Work out the finished part from the listing and answer in its coordinate system (mm). Face numbers are marked on the shaded views. A direction names the side the tool comes from. Round coordinates to 2 decimals unless told otherwise and drop trailing zeros. Order: outer loops, then holes, each group sorted by start corner. A loop starts at its lowest first (then second) coordinate and runs counter-clockwise, first axis right, second up. Notation, with made-up numbers: (-12.5, 27) -> (8.5, 27) arc R9 ccw to (8.5, 31) -> close; hole circle Ø7 at (50, 41). An arc over 180 degrees is marked (long way). Use a Markdown table: item, result. Add a question column.
Item 1: A cutting plane is placed at C-C, the plane z = 15. Determine the outline of the cut face in (x, y).
Item 2: A cutting plane is placed at A-A, the plane y = 0. Determine the outline of the cut face in (x, z), plus the area to 3 significant figures.
Item 3: Find the intervals of material crossed by L1, parallel to Z at x = 2, y = -0.75; L2, parallel to X at y = 5.25, z = 17.5; L3, parallel to Y at x = -6.75, z = 5.75, in increasing order. Write a range as [from, to].
Item 4: A tool of negligible diameter and unlimited length cuts with its end or side. For the marked faces 1, 2 and 3, from which of +Z, -Z, +X, -X, +Y, -Y can it reach the whole face along a straight path? Write none if from no direction.
Item 5: Flat-ended cylindrical pins translate along their axes: P1, Ø1.5, axis at y = -1.5, z = 12.5, coming from the +X side; P2, Ø2, axis at x = -3, z = -0.5, coming from the -Y side; P3, Ø2, axis at x = 2.5, z = 8.5, coming from the +Y side. Find the tip coordinate at first contact, or state that the pin passes through.
from build123d import *

# Parameters (mm, degrees)
BOSS_EXTRUDE1_START = 2
SKETCH2_R           = 1.25
BOSS_EXTRUDE1_DEPTH = 2


with BuildPart() as part:
    # Sketch1 → Revolve1 (revolve)
    with BuildSketch(Plane(origin=(0, 0, 0), x_dir=(1, 0, 0), z_dir=(0, 1, 0))):
        Polygon((1.25, 1.9), (0, 1.9), (0, -22.7), (0.8476, -22.7), (1, -22.5476), (1, -18.7), (9.125906359, -18.7), (10.5, -16.32), (10.5, -2.840563324), (5.58, 0), (2.75, 0), (2.75, 0.95), (1.25, 0.95), align=None)
    revolve(axis=Axis((0, 0, -1.9), (0, 0, 1)))

    # Sketch2 → Boss-Extrude1 (add)
    with BuildSketch(Plane(origin=(0, 0, -1.9), x_dir=(-1, 0, 0), z_dir=(0, 0, -1)).offset(BOSS_EXTRUDE1_START)):
        with Locations(Location((0, 0, 0), (0, 0, 180))):
            Circle(SKETCH2_R)
    extrude(amount=-BOSS_EXTRUDE1_DEPTH)


solid = part.part
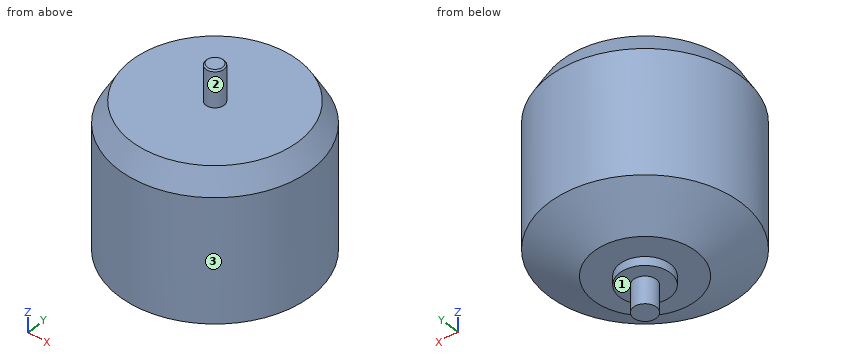
Reported:
| question | item | result |
|---|---|---|
| 1 | outline | circle Ø21 at (0, 0) |
| 2 | outline | (-10.5, 2.84) -> (-5.58, 0) -> (-2.75, 0) -> (-2.75, -0.95) -> (-1.25, -0.95) -> (-1.25, -3.9) -> (1.25, -3.9) -> (1.25, -0.95) -> (2.75, -0.95) -> (2.75, 0) -> (5.58, 0) -> (10.5, 2.84) -> (10.5, 16.32) -> (9.13, 18.7) -> (1, 18.7) -> (1, 22.55) -> (0.85, 22.7) -> (-0.85, 22.7) -> (-1, 22.55) -> (-1, 18.7) -> (-9.13, 18.7) -> (-10.5, 16.32) -> close |
| 2 | area | 396 mm² |
| 3 | L1 | [-0.95, 18.7] |
| 3 | L2 | [-8.3, 8.3] |
| 3 | L3 | [-8.04, 8.04] |
| 4 | face 1 | -Z |
| 4 | face 2 | +Z |
| 4 | face 3 | +Z, -Z |
| 5 | P1 | x = 10.47 |
| 5 | P2 | y = -5.77 |
| 5 | P3 | y = 10.39 |
